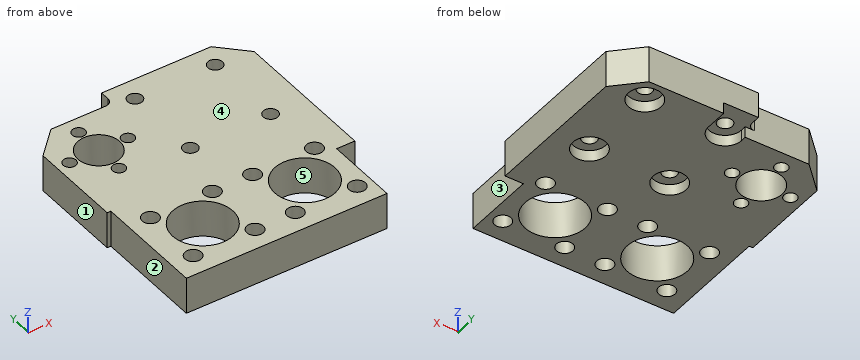
Autodesk Inventor part; units mm, degrees
ref_plane "YZ Plane" through (0, 0, 0) normal (1, 0, 0) x (0, 1, 0)
ref_plane "XZ Plane" through (0, 0, 0) normal (0, 1, 0) x (-1, 0, 0)
ref_plane "XY Plane" through (0, 0, 0) normal (0, 0, 1) x (1, 0, 0)
sketch "Sketch1" plane through (0, 0, 0) normal (0, 0, 1) x (1, 0, 0)
  line L0 (-32.5, 33.5) -> (32.5, 33.5)
  line L1 (32.5, 33.5) -> (32.5, -33.5)
  line L2 (32.5, -33.5) -> (-32.5, -33.5)
  line L3 (-32.5, -33.5) -> (-32.5, 33.5)
  point P0 (0, 0)
  point P1 (0, 33.5)
  point P2 (-32.5, 0)
  dimension "d0" = 65
  dimension "d1" = 67
extrude "Extrusion1" add sketch "Sketch1" along normal blind 10
sketch "Sketch5" plane through (0, 0, 0) normal (0, 0, -1) x (-1, 0, 0)
  circle A0 centre (-0.5, 27.5) radius 2
  circle A1 centre (-0.5, 5.5) radius 2
  line L0 (32.5, 33.5) -> (32.5, -33.5)
  line L1 (-32.5, 33.5) -> (32.5, 33.5)
  circle A2 centre (-22.5, 5.5) radius 2
  circle A3 centre (-22.5, 27.5) radius 2
  line L2 (-32.5, -33.5) -> (-32.5, 33.5)
  point P0 (0, 0)
  dimension "d30" = 6
  dimension "d31" = 4
  dimension "d32" = 22
  dimension "d50" = 22
  dimension "d51" = 10
hole "Hole1" at (0.5, 5.5, 0) at (0.5, 27.5, 0) at (22.5, 5.5, 0) at (22.5, 27.5, 0) direction (0, 0, 1) diameter 4 depth 11 tip angle 118 counterbore diameter 9 counterbore depth 3
sketch "Sketch6" plane through (0, 0, 0) normal (0, 0, -1) x (-1, 0, 0)
  line L0 (4, 23) -> (-5, 23)
  line L1 (-5, 23) -> (-5, 33.5)
  line L2 (-5, 33.5) -> (4, 33.5)
  line L3 (4, 33.5) -> (4, 23)
  line L4 (-32.5, 33.5) -> (32.5, 33.5)
  circle A0 centre (-0.5, 27.5) radius 4.5
  line L5 (6, 29) -> (4, 29)
  line L6 (4, 29) -> (4, 33.5)
  line L7 (4, 33.5) -> (6, 33.5)
  line L8 (6, 33.5) -> (6, 29)
  point P0 (0, 0)
  point P1 (-5, 27.5)
  point P2 (4, 27.5)
  point P3 (6, 33.5)
  point P4 (4, 33.5)
  point P5 (4, 29)
  dimension "d77" = 2
  dimension "d78" = 4.5
extrude "Extrusion4" cut sketch "Sketch6" against normal up to surface (3 mm away) contours A0 L1 L2 L3 | L3 L4 L8 L5
sketch "Sketch7" plane through (0, 0, 0) normal (0, 0, -1) x (-1, 0, 0)
  circle A0 centre (17, 16.5) radius 5.75
  circle A1 centre (17, 16.5) radius 8 construction
  circle A2 centre (17, 24.5) radius 1.75
  line L0 (6, 33.5) -> (32.5, 33.5)
  line L1 (32.5, 33.5) -> (32.5, -33.5)
  circle A3 centre (9, 16.5) radius 1.75
  circle A4 centre (17, 8.5) radius 1.75
  circle A5 centre (25, 16.5) radius 1.75
  line L2 (6, 33.5) -> (-5, 33.5)
  line L3 (-32.5, -33.5) -> (-32.5, 33.5)
  point P0 (4, 33.5)
  point P1 (25.5, 33.5)
  point P2 (32.5, 26.5)
  point P3 (-25.5, 33.5)
  point P4 (-32.5, 26.5)
  dimension "d55" = 16
  dimension "d52" = 11.5
  dimension "d54" = 3.5
  dimension "d61" = 360
  dimension "d65" = 17
  dimension "d66" = 49.5
extrude "Extrusion5" cut sketch "Sketch7" against normal through all
sketch "Sketch8" plane through (0, 0, 0) normal (0, 0, -1) x (-1, 0, 0)
  line L0 (32.5, -33.5) -> (-32.5, -33.5)
  line L1 (32.5, -33.5) -> (27.5, -33.5)
  line L2 (27.5, -33.5) -> (27.5, -3.5)
  line L3 (27.5, -3.5) -> (32.5, -3.5)
  line L4 (32.5, -3.5) -> (32.5, -33.5)
  line L5 (-27.5, -33.5) -> (-32.5, -33.5)
  line L6 (-32.5, -33.5) -> (-32.5, -13.5)
  line L7 (-32.5, -13.5) -> (-27.5, -13.5)
  line L8 (-27.5, -13.5) -> (-27.5, -33.5)
  line L9 (32.5, -33.5) -> (-32.5, -33.5)
  line L10 (-32.5, -33.5) -> (-32.5, 33.5)
  line L11 (32.5, 33.5) -> (32.5, -33.5)
  point P0 (0, 0)
  point P1 (-32.5, 26.5)
  point P2 (32.5, 26.5)
  dimension "d67" = 5
  dimension "d68" = 5
  dimension "d69" = 30
  dimension "d72" = 20
extrude "Extrusion6" cut sketch "Sketch8" against normal through all
sketch "Sketch9" plane through (0, 0, 10) normal (0, 0, 1) x (1, 0, 0)
  line L0 (-30.5, 33) -> (-7.5, 33)
  line L1 (-32.5, 33.5) -> (-4.5, 33.5)
  line L2 (-4.5, 33.5) -> (-4.5, 29)
  line L3 (-4.5, 29) -> (-32.5, 29)
  line L4 (-32.5, 29) -> (-32.5, 33.5)
  line L5 (-32.5, 33.5) -> (-32.5, -3.5)
  line L6 (32.5, 33.5) -> (-32.5, 33.5)
  point P0 (0, 0)
  point P1 (-32.5, 26.5)
  point P2 (25.5, 33.5)
  point P3 (-25.5, 33.5)
  dimension "d73" = 4
  dimension "d74" = 3
extrude "Extrusion7" cut sketch "Sketch9" against normal through all
sketch "Sketch10" plane through (0, 0, 0) normal (0, 0, -1) x (-1, 0, 0)
  circle A0 centre (-15, -19) radius 4
  circle A1 centre (-23.4853, -10.5147) radius 1.7
  circle A2 centre (-6.5147, -10.5147) radius 1.7
  circle A3 centre (-6.5147, -27.4853) radius 1.7
  circle A4 centre (-23.4853, -27.4853) radius 1.7
  circle A5 centre (-15, -19) radius 7.5
  line L0 (-25.1274, -6.5) -> (-4.8726, -6.5)
  line L1 (-4.8726, -6.5) -> (-2.5, -8.8726)
  line L2 (-2.5, -8.8726) -> (-2.5, -29.1274)
  line L3 (-2.5, -29.1274) -> (-4.8726, -31.5)
  line L4 (-4.8726, -31.5) -> (-25.1274, -31.5)
  line L5 (-25.1274, -31.5) -> (-27.5, -29.1274)
  line L6 (-27.5, -29.1274) -> (-27.5, -8.8726)
  line L7 (-27.5, -8.8726) -> (-25.1274, -6.5)
  circle A6 centre (13, -19) radius 4
  circle A7 centre (21.4853, -10.5147) radius 1.7
  circle A8 centre (21.4853, -27.4853) radius 1.7
  circle A9 centre (4.5147, -27.4853) radius 1.7
  circle A10 centre (4.5147, -10.5147) radius 1.7
  circle A11 centre (13, -19) radius 7.5
  line L8 (25.5, -8.8726) -> (25.5, -29.1274)
  line L9 (25.5, -29.1274) -> (23.1274, -31.5)
  line L10 (23.1274, -31.5) -> (2.8726, -31.5)
  line L11 (2.8726, -31.5) -> (0.5, -29.1274)
  line L12 (0.5, -29.1274) -> (0.5, -8.8726)
  line L13 (0.5, -8.8726) -> (2.8726, -6.5)
  line L14 (2.8726, -6.5) -> (23.1274, -6.5)
  line L15 (23.1274, -6.5) -> (25.5, -8.8726)
  circle A12 centre (-15, -19) radius 8.25
  circle A13 centre (13, -19) radius 8.25
  circle A14 centre (21.4853, -27.4853) radius 2.25
  circle A15 centre (4.5147, -27.4853) radius 2.25
  circle A16 centre (21.4853, -10.5147) radius 2.25
  circle A17 centre (4.5147, -10.5147) radius 2.25
  circle A18 centre (-6.5147, -27.4853) radius 2.25
  circle A19 centre (-23.4853, -27.4853) radius 2.25
  circle A20 centre (-23.4853, -10.5147) radius 2.25
  circle A21 centre (-6.5147, -10.5147) radius 2.25
  point P0 (0, 0)
  dimension "d79" = 16.5
  dimension "d80" = 16.5
  dimension "d81" = 4.5
  dimension "d82" = 4.5
  dimension "d83" = 4.5
  dimension "d84" = 4.5
  dimension "d85" = 4.5
  dimension "d86" = 4.5
  dimension "d87" = 4.5
  dimension "d88" = 4.5
extrude "Extrusion8" cut sketch "Sketch10" against normal through all contours A0 | A1 | A2 | A3 | A4 | A5 | A6 | A7 | A8 | A9 | A10 | A11 | A12 | A13 | A14 | A15 | A16 | A17 | A18 | A19 | A20 | A21
move faces "Move1" translate (4, 0, 0) faces at (-32.5, 18.1667, 3.3333)
chamfer "Chamfer2" distance 7 angle 45 2 edges at (-28.5, 29, 5) (32.5, 33.5, 5)
fillet "Fillet1" radius 2 1 edges at (-4.5, 29, 6.5)
equation "\"d50\" = d32"
equation "\"d68\" = d67"
equation "\"d80\" = d79"
equation "\"BendRadius\" = Thickness"
equation "\"BendReliefWidth\" = Thickness"
equation "\"BendReliefDepth\" = 0.5 * Thickness"
equation "\"CornerReliefSize\" = 4 * Thickness"
equation "\"MinimumRemnant\" = 2 * Thickness"
equation "\"TransitionRadius\" = BendRadius"
equation "\"JacobiRadiusSize\" = Thickness"
equation "\"GapSize\" = Thickness"
properties part number "0008-10-001" material "ABS Plastic"
Could you check a few things on this model? Use its own coordinates, in mm. Face numbers are marked on the shaded views. A direction names the side the tool comes from. Round coordinates to 2 decimals unless told otherwise and drop trailing zeros. Loops run counter-clockwise (first coordinate to the right, second up) from the corner with the lowest first, then second, coordinate; pieces in that order, holes last.
Q1. I want a section at D-D (y = -24). Write out the boundary of the cut face in (x, z).
Q2. Please list where these lines run through material, in increasing order: L1, parallel to X at y = 17.5, z = 6.5; L2, parallel to X at y = 4.5, z = 0.5; L3, parallel to X at y = -4.5, z = 3.
Q3. I want a section at C-C (y = 8.5). Write out the boundary of the cut face in (x, z), and give its area (3 significant figures).
Q4. Thinking about a two-plate mould opening in X: for the marked faces 3, 4 and 5, which applies, pulls with the +X half, pulls with the -X half, needs draft (parallel to the pull), parting line crosses it, or undercut?
Q5. On a 3-axis mill with a long thin cutter (end or side, diameter ignored), from which of +Z, -Z, +X, -X, +Y, -Y can I reach the whole of each face in a straight line? I mean the marked faces 1 and 2. Say none if no direction works.
Q6. I want a section at A-A (x = 15). Write out the boundary of the cut face in (y, z).
Q7. For P1, Ø7, axis at x = -21.49, y = -10.51, coming from the +Z side; P2, Ø13, axis at x = -13, y = -19, coming from the +Z side; P3, Ø1.2, axis at y = 32, z = 7, coming from the -X side; P4, Ø4, axis at x = 30, z = 6, coming from the -Y side, each with a flat end and sliding along its axis, tell me the tip position at first contact or that it passes through.
Q8. I want a section at B-B (x = -13). Write out the boundary of the cut face in (y, z), and give its area (3 significant figures).
Answer below:
1. outline: (-27.5, 0) - (-19.56, 0) - (-19.56, 10) - (-27.5, 10) - close; (-6.44, 0) - (8.44, 0) - (8.44, 10) - (-6.44, 10) - close; (21.56, 0) - (27.5, 0) - (27.5, 10) - (21.56, 10) - close
2. L1: x = -28.5 to -26.44, -23.56 to -22.66, -11.34 to -10.44, -7.56 to 32.5
2. L2: x = -28.5 to -3.89, 4.89 to 18.11, 26.89 to 32.5
2. L3: x = -27.5 to 32.5
3. outline: (-28.5, 0) - (-18.75, 0) - (-18.75, 10) - (-28.5, 10) - close; (-15.25, 0) - (-2.85, 0) - (-2.85, 3) - (3.85, 3) - (3.85, 0) - (19.15, 0) - (19.15, 3) - (25.85, 3) - (25.85, 0) - (32.5, 0) - (32.5, 10) - (-15.25, 10) - close
3. area: 535 mm2
4. face 3: pulls with the +X half
4. face 4: needs draft
4. face 5: undercut
5. face 1: +Z, -Z, -X, +Y, -Y
5. face 2: +Z, -Z, -X, -Y
6. outline: (-33.5, 0) - (-27.25, 0) - (-27.25, 10) - (-33.5, 10) - close; (-10.75, 0) - (33.5, 0) - (33.5, 10) - (-10.75, 10) - close
7. P1: stops at z = 10
7. P2: passes through
7. P3: stops at x = -4.5
7. P4: stops at y = -13.5
8. outline: (-33.5, 0) - (-27.25, 0) - (-27.25, 10) - (-33.5, 10) - close; (-10.75, 0) - (12.37, 0) - (12.37, 10) - (-10.75, 10) - close; (20.63, 0) - (29, 0) - (29, 10) - (20.63, 10) - close
8. area: 377 mm2
